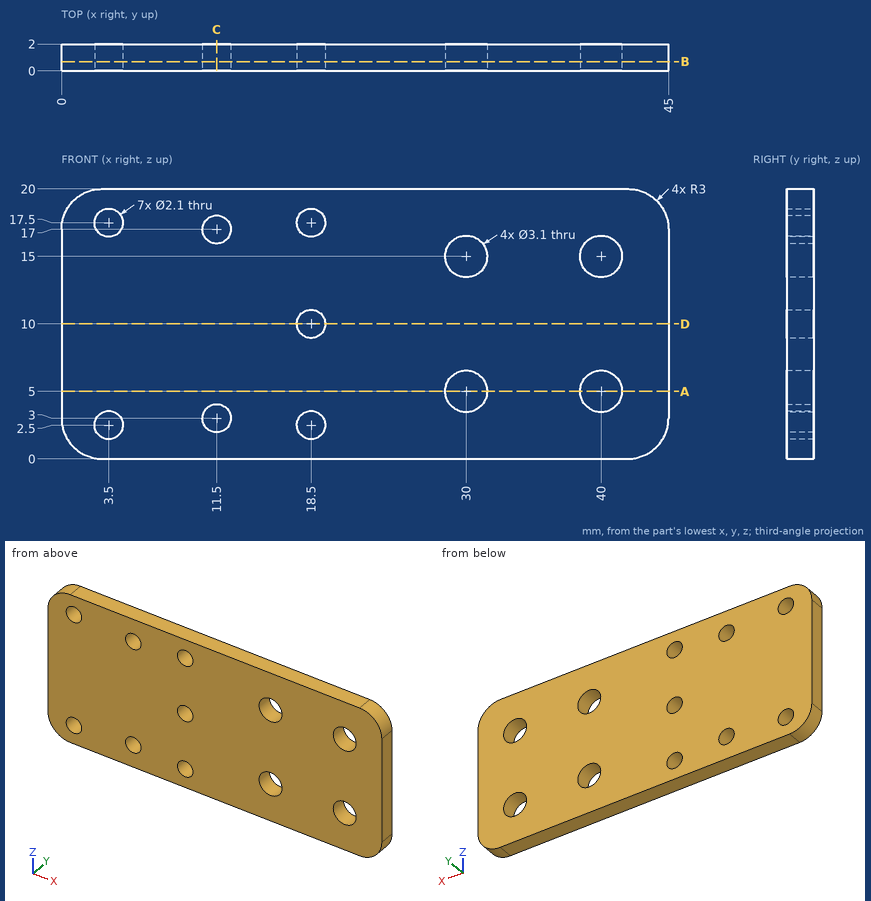
Job drawing, mm, ordinate dimensions from the low corner. One solid piece. Coordinates: 2 decimals unless noted, no trailing zeros. Loops run counter-clockwise (first coordinate to the right, second up) from the corner with the lowest first, then second, coordinate; pieces in that order, holes last. Notation, with made-up numbers: (45, -6) - (57, -6) arc R27 cw to (57, 30) - close; hole circle Ø4 at (-40, 7.25). An arc over 180 degrees is marked (long way). Answer as a JSON object with one key per item and string values. Group by question number.
(1) Cut at C-C (x = 11.5). Give the cut face in (y, z), then the cut area to 3 significant figures.
(2) Cut at A-A (z = 5). Give the cut face in (x, y), then the cut area to 3 significant figures.
(3) Cut at B-B (y = 0.7). State how many separate pieces and enclosed holes the cut face has, then the cut area to 3 significant figures.
(4) Probe line 1 along X through (y, z) = (1.8, 15); line 2 along X through (y, z) = (1.65, 18.25); line 3 along X through (y, z) = (1.45, 17.5). List the from-to ranges inside material, lowest first.
(5) Cut at D-D (z = 10). Give the cut face in (x, y).
(6) Flat gauge pin, fed straight in: pin 1 (1.3 mm diameter, centred on x = 18.5, z = 2.5, fed in from -Y). Where does the tip first touch, or does it go through?
Geometry says:
{
 "1": {"outline": "(0, 0) - (2, 0) - (2, 1.95) - (0, 1.95) - close; (0, 4.05) - (2, 4.05) - (2, 15.95) - (0, 15.95) - close; (0, 18.05) - (2, 18.05) - (2, 20) - (0, 20) - close", "area": "31.6 mm^2"},
 "2": {"outline": "(0, 0) - (28.45, 0) - (28.45, 2) - (0, 2) - close; (31.55, 0) - (38.45, 0) - (38.45, 2) - (31.55, 2) - close; (41.55, 0) - (45, 0) - (45, 2) - (41.55, 2) - close", "area": "77.6 mm^2"},
 "3": {"separate pieces": "1", "enclosed holes": "11", "area": "838 mm^2"},
 "4": {"line 1": "x = 0 to 28.45, 31.55 to 38.45, 41.55 to 45", "line 2": "x = 0.27 to 2.77, 4.23 to 17.77, 19.23 to 44.73", "line 3": "x = 0.04 to 2.45, 4.55 to 10.58, 12.42 to 17.45, 19.55 to 44.96"},
 "5": {"outline": "(0, 0) - (17.45, 0) - (17.45, 2) - (0, 2) - close; (19.55, 0) - (45, 0) - (45, 2) - (19.55, 2) - close"},
 "6": {"pin 1": "passes through"}
}
